```python
from build123d import *

# Parameters (mm, degrees)
BOSS_EXTRUDE1_DEPTH        = 4.5
BOSS_EXTRUDE1_DEPTH_BACK   = 4.5
F_4_4_4_4_DIAMETER_HOLE1_D = 4.4
CUT_EXTRUDE1_START         = -8
SKETCH7_R                  = 3.5
CUT_EXTRUDE1_DEPTH         = 18


with BuildPart() as part:
    # Sketch1 → Boss-Extrude1 (new body, two sides)
    with BuildSketch(Plane(origin=(0, 0, 0), x_dir=(1, 0, 0), z_dir=(0, 1, 0))) as boss_extrude1_sk:
        with BuildLine():
            Line((-27.5, 0), (-17.5, 0))
            ThreePointArc((-17.5, 0), (0, 17.5), (17.5, 0))
            Line((17.5, 0), (27.5, 0))
            ThreePointArc((27.5, 0), (0, 27.5), (-27.5, 0))
        make_face()
    extrude(amount=BOSS_EXTRUDE1_DEPTH)
    extrude(boss_extrude1_sk.sketch, amount=-BOSS_EXTRUDE1_DEPTH_BACK)

    # 4.4 _4.4_ Diameter Hole1 (through all)
    with Locations(Plane(origin=(22.5, 0, 0), x_dir=(1, 0, 0), z_dir=(0, 0, 1))):
        with Locations((0, 0), (-45, 0)):
            Hole(F_4_4_4_4_DIAMETER_HOLE1_D / 2)

    # Sketch7 → Cut-Extrude1 (cut)
    with BuildSketch(Plane.XY.offset(CUT_EXTRUDE1_START)):
        with Locations((-22.5, 0)):
            Circle(SKETCH7_R)
        with Locations((22.5, 0)):
            Circle(SKETCH7_R)
    extrude(amount=-CUT_EXTRUDE1_DEPTH, mode=Mode.SUBTRACT)


solid = part.part
```
The listing builds one solid part. Answer for the finished solid, in the listing's coordinates (mm). A direction names the side the tool comes from. Give positions to 0.01 mm unless a question says otherwise; leave off trailing zeros. Loops run counter-clockwise (first coordinate to the right, second up) from the corner with the lowest first, then second, coordinate; pieces in that order, holes last. Notation, with made-up numbers: (-15.75, 85) - (39.25, 85) arc R16 ccw to (39.25, 92) - close; hole circle Ø1 at (-7, 7.5). An arc over 180 degrees is marked (long way). Return JSON: item names as keys, results as strings. Group by question number.
1. Find section B-B (x = -22). Write down the section's boundary in (y, z).
2. Which of the six approach directions +Z, -Z, +X, -X, +Y, -Y give full straight-line access (tool end or side, diameter ignored) to faces 4 (the cylindrical face through (19, 0, -13)), 5 (the flat face through (-25, 0, 0))?
3. Find section D-D (z = -19). Write down the section's boundary in (x, y).
4. Given pin 1 Ø4 at (y, z) = (2.5, -24.5) entering from +X; pin 2 Ø4 at (x, y) = (2, -1) entering from +Z; pin 3 Ø3.5 at (x, y) = (24, -0.5) entering from -Z, each flat-ended and moving along its own axis, determine where each tip first touches the part or whether it passes through.
5. Find section A-A (y = -1). Write down the section's boundary in (x, z), then the cut area to 3 significant figures.
6. Straight lines are drawn through the part: line 1 (X direction, y = -0.25, z = -6.75); line 2 (Y direction, x = 22.5, z = -5); line 3 (Z direction, x = 21, y = -2.5). For each, find the intervals that lie inside material, in ascending order. Write a range as [from, to].
7. Determine the mould class of faces 1 (the flat face through (0, 4.5, -20)), 2 (the flat face through (20, 0, 0)), 3 (the cylindrical face through (-24.532, -0.843, -4.056)) for opening direction Y: pulls with the +Y half, pulls with the -Y half, needs draft (parallel to the pull), parting line crosses it, or undercut.
Verdict:
{
 "1": {"outline": "(-4.5, -16.5) - (-3.46, -16.5) - (-3.46, -8) - (-2.14, -8) - (-2.14, 0) - (-4.5, 0) - close; (2.14, -8) - (3.46, -8) - (3.46, -16.5) - (4.5, -16.5) - (4.5, 0) - (2.14, 0) - close"},
 "2": {"face 4": "-Z", "face 5": "+Z, +X, -X, +Y, -Y"},
 "3": {"outline": "(-19.88, -4.5) - (19.88, -4.5) - (19.88, -2.32) arc R3.5 cw to (19.88, 2.32) - (19.88, 4.5) - (-19.88, 4.5) - (-19.88, 2.32) arc R3.5 cw to (-19.88, -2.32) - close"},
 "4": {"pin 1": "stops at x = 15.81", "pin 2": "stops at z = -17.04", "pin 3": "stops at z = -8"},
 "5": {"outline": "(-27.5, 0) arc R27.5 ccw to (-25.85, -9.37) - (-25.85, -8) - (-24.46, -8) - (-24.46, 0) - close; (-20.54, -8) - (-19.15, -8) - (-19.15, -19.74) arc R27.5 ccw to (19.15, -19.74) - (19.15, -8) - (20.54, -8) - (20.54, 0) - (17.5, 0) arc R17.5 cw to (-17.5, 0) - (-20.54, 0) - close; (24.46, -8) - (25.85, -8) - (25.85, -9.37) arc R27.5 ccw to (27.5, 0) - (24.46, 0) - close", "area": "545 mm^2"},
 "6": {"line 1": "x = [-26.66, -24.69], [-20.31, -16.15], [16.15, 20.31], [24.69, 26.66]", "line 2": "y = [-4.5, -2.2], [2.2, 4.5]", "line 3": "z = [-8, 0]"},
 "7": {"face 1": "pulls with the +Y half", "face 2": "needs draft", "face 3": "undercut"}
}
